Can you work these out from the drawing? Everything is in mm from the part's minimum corner. Give positions to 0.01 mm unless a question says otherwise; leave off trailing zeros. Loops run counter-clockwise (first coordinate to the right, second up) from the corner with the lowest first, then second, coordinate; pieces in that order, holes last. Notation, with made-up numbers: (75.5, -10) - (89.5, -10) arc R17 ccw to (89.5, 1) - close; hole circle Ø5 at (0, -14.5). An arc over 180 degrees is marked (long way). One line per item, written item: value. Start each with the question number.
Q1. I want a section at A-A (z = 0.45). Please give me the cut outline in (x, y).
Q2. I'm going to push flat-ended pins straight in: P1, Ø0.5, axis at y = 13, z = 0.5, coming from the +X side; P2, Ø0.5, axis at x = 24, z = 0.5, coming from the -Y side. Where does each tip first touch, or does it pass through?
Q3. I want a section at C-C (x = 6.5). Please give me the cut outline in (y, z).
Q4. I want a section at B-B (y = 24). Please give me the cut outline in (x, z).
Q5. If I drill on line 1 (Y direction, x = 6.5, z = 0.6); line 2 (X direction, y = 7, z = 0.6), over which ranges is the centre line in solid material (lowest first)? Write a range as from..to.
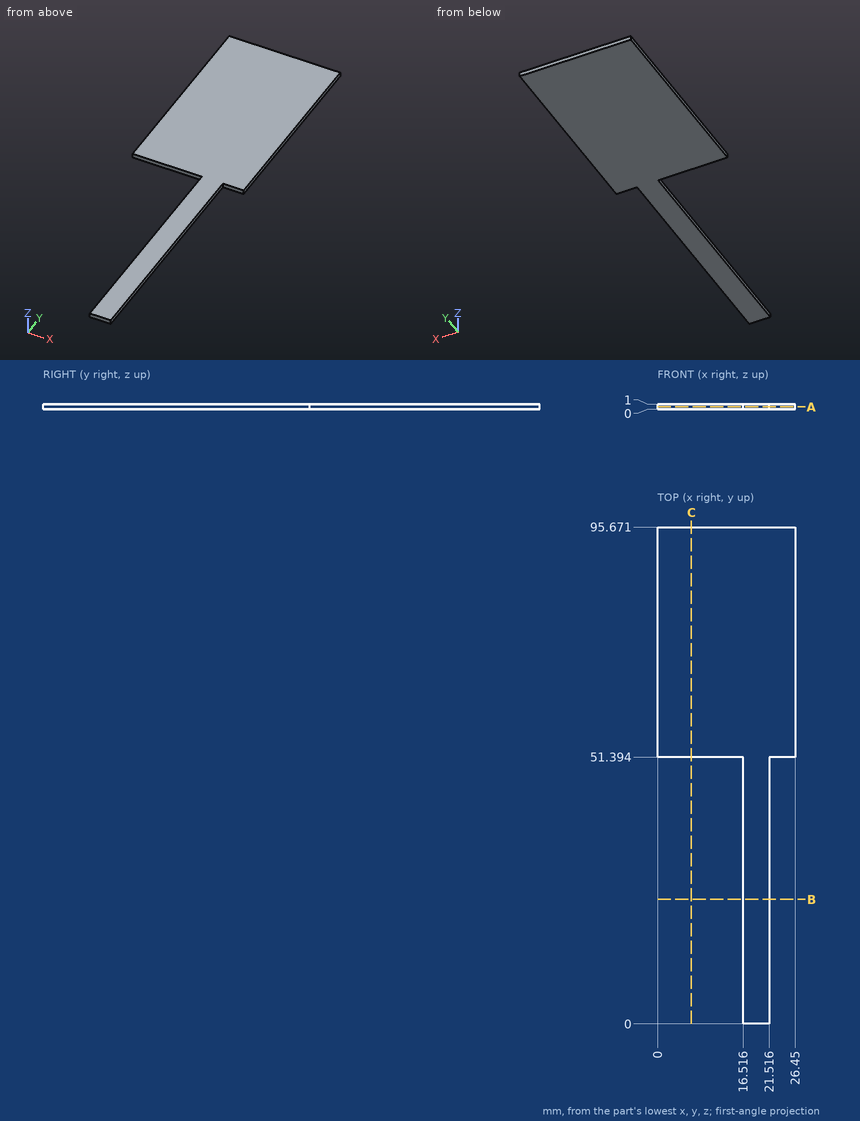
Worked answers:
1. outline: (0, 51.39) - (16.52, 51.39) - (16.52, 0) - (21.52, 0) - (21.52, 51.39) - (26.45, 51.39) - (26.45, 95.67) - (0, 95.67) - close
2. P1: stops at x = 21.52
2. P2: stops at y = 51.39
3. outline: (51.39, 0) - (95.67, 0) - (95.67, 1) - (51.39, 1) - close
4. outline: (16.52, 0) - (21.52, 0) - (21.52, 1) - (16.52, 1) - close
5. line 1: y = 51.39..95.67
5. line 2: x = 16.52..21.52
